Autodesk Inventor part; units mm, degrees
ref_plane "YZ Plane" through (0, 0, 0) normal (1, 0, 0) x (0, 1, 0)
ref_plane "XZ Plane" through (0, 0, 0) normal (0, 1, 0) x (-1, 0, 0)
ref_plane "XY Plane" through (0, 0, 0) normal (0, 0, 1) x (1, 0, 0)
sketch "スケッチ1" plane through (0, 0, 0) normal (0, 1, 0) x (-1, 0, 0)
  line L0 (-6, -13) -> (6, -13)
  line L1 (6, -13) -> (6, 13)
  line L2 (6, 13) -> (-6, 13)
  line L3 (-6, 13) -> (-6, -13)
  line L4 (-6, -13) -> (6, 13) construction
  line L5 (6, -13) -> (-6, 13) construction
  line L6 (6, 13) -> (-6, 13)
  line L7 (-6, 13) -> (-6, 5)
  line L8 (-6, 5) -> (6, 5)
  line L9 (6, 5) -> (6, 13)
  point P0 (0, 0)
  point P1 (0, 13)
  point P2 (-6, 13)
  point P3 (6, 5)
  dimension "d0" = 12
  dimension "d1" = 26
  dimension "d26" = 12
  dimension "d27" = 8
extrude "押し出し1" add sketch "スケッチ1" against normal blind 3 contours L3 L8 L1 L0
sketch "スケッチ5" plane through (0, 0, 0) normal (1, 0, 0) x (0, 1, 0)
  line L0 (-3, 5) -> (-3, -13)
  line L1 (-3, 5) -> (-3, 13)
  line L2 (-1.6051, 5) -> (-12.6984, 24.2141)
  line L3 (-12.6984, 24.2141) -> (-17.6984, 24.2141)
  line L4 (-16.3866, 0) -> (-3, 0)
  line L5 (0, 5) -> (-3, 5)
  line L6 (-17.6984, 24.2141) -> (-22.1813, 21.6259)
  line L7 (-22.1813, 21.6259) -> (-16.3866, 0)
  line L8 (-12.6984, 24.2141) -> (-8.3683, 26.7141) construction
  line L9 (-8.3683, 26.7141) -> (-7.6183, 25.4151) construction
  circle A0 centre (-7.6183, 25.4151) radius 1 construction
  line L10 (36.5, 48) -> (-6.3683, 23.25) construction
  line L11 (0, 13) -> (36.5, 13) construction
  line L12 (0, -13) -> (0, 5)
  line L13 (-3, 5) -> (-1.6051, 5)
  point P0 (0, 0)
  dimension "d28" = 8
  dimension "d29" = 120
  dimension "d31" = 5
  dimension "d32" = 5
  dimension "d35" = 5
  dimension "d36" = 150
  dimension "d37" = 75
  dimension "d47" = 5
  dimension "d48" = 1.5
  dimension "d49" = 2
  dimension "d50" = 2.5
  dimension "d51" = 49.5
  dimension "d53" = 8
  dimension "d54" = 36.5
  dimension "d55" = 35
extrude "押し出し5" add sketch "スケッチ5" against normal blind 4
sketch "スケッチ6" plane through (-4, 0, 0) normal (-1, 0, 0) x (0, 0, 1)
  line L0 (0, -3) -> (0, -16.3866)
  line L1 (0, -16.3866) -> (21.6259, -22.1813)
  line L2 (21.6259, -22.1813) -> (24.2141, -17.6984)
  line L3 (24.2141, -17.6984) -> (24.2141, -12.6984)
  line L4 (24.2141, -12.6984) -> (5, -1.6051)
  line L5 (0, -3) -> (5, -3)
  line L6 (19.884, -10.1984) -> (14.1259, -20.1716)
  line L7 (24.2141, -12.6984) -> (5.604, -1.9538)
  line L8 (5, -3) -> (5, -1.6051)
  point P0 (0, 0)
  dimension "d38" = 5
extrude "押し出し6" add sketch "スケッチ6" along normal blind 6 contours L6 L4 L3 L2 L1
mirror "ミラー3" about plane through (0, -11.8932, 12.1071) normal (1, 0, 0) of "押し出し5", "押し出し6"
sketch "スケッチ7" plane through (0, 0, 0) normal (0, 1, 0) x (1, 0, 0)
  circle A0 centre (4, -3) radius 1
  circle A1 centre (-4, 11) radius 1
  circle A2 centre (0, 0) radius 0.8
  circle A3 centre (0, 8) radius 0.8
  circle A4 centre (-4, 4) radius 0.8
  circle A5 centre (4, 4) radius 0.8
  circle A6 centre (4, 11) radius 1
  circle A7 centre (-4, -3) radius 1
  line L0 (6, -8) -> (6, -10)
  line L1 (30, -13) -> (9, -13)
  line L2 (33, -9.25) -> (33, -10)
  arc A8 (30, 6.25) -> (30, -6.25) centre (30, 0) ccw
  line L3 (33, 10) -> (33, 9.25)
  line L4 (-30, 13) -> (30, 13)
  line L5 (-33, -10) -> (-33, -9.25)
  arc A9 (-30, -6.25) -> (-30, 6.25) centre (-30, 0) ccw
  line L6 (-33, 9.25) -> (-33, 10)
  line L7 (-9, -13) -> (-30, -13)
  line L8 (-6, -10) -> (-6, -8)
  line L9 (-3, -5) -> (3, -5)
  line L10 (21.75, 7.5) -> (21.75, -7.5)
  line L11 (18.75, -10.5) -> (14, -10.5)
  line L12 (11, -7.5) -> (11, 7.5)
  line L13 (14, 10.5) -> (18.75, 10.5)
  circle A10 centre (9, 10.5) radius 0.85
  circle A11 centre (30, -10.5) radius 0.85
  circle A12 centre (-30, -10.5) radius 0.85
  circle A13 centre (-9, 10.5) radius 0.85
  circle A14 centre (-30, 10.5) radius 0.85
  circle A15 centre (-9, -10.5) radius 0.85
  circle A16 centre (9, -10.5) radius 0.85
  circle A17 centre (30, 10.5) radius 0.85
  line L14 (-11, 7.5) -> (-11, -7.5)
  line L15 (-14, -10.5) -> (-18.75, -10.5)
  line L16 (-21.75, -7.5) -> (-21.75, 7.5)
  line L17 (-18.75, 10.5) -> (-14, 10.5)
  arc A18 (-30, 13) -> (-33, 10) centre (-30, 10) ccw
  arc A19 (-33, 9.25) -> (-30, 6.25) centre (-30, 9.25) ccw
  arc A20 (-30, -6.25) -> (-33, -9.25) centre (-30, -9.25) ccw
  arc A21 (-33, -10) -> (-30, -13) centre (-30, -10) ccw
  arc A22 (-9, -13) -> (-6, -10) centre (-9, -10) ccw
  arc A23 (-3, -5) -> (-6, -8) centre (-3, -8) ccw
  arc A24 (6, -8) -> (3, -5) centre (3, -8) ccw
  arc A25 (6, -10) -> (9, -13) centre (9, -10) ccw
  arc A26 (30, -13) -> (33, -10) centre (30, -10) ccw
  arc A27 (33, -9.25) -> (30, -6.25) centre (30, -9.25) ccw
  arc A28 (30, 6.25) -> (33, 9.25) centre (30, 9.25) ccw
  arc A29 (33, 10) -> (30, 13) centre (30, 10) ccw
  arc A30 (-14, -10.5) -> (-11, -7.5) centre (-14, -7.5) ccw
  arc A31 (-21.75, -7.5) -> (-18.75, -10.5) centre (-18.75, -7.5) ccw
  arc A32 (-18.75, 10.5) -> (-21.75, 7.5) centre (-18.75, 7.5) ccw
  arc A33 (-11, 7.5) -> (-14, 10.5) centre (-14, 7.5) ccw
  arc A34 (18.75, -10.5) -> (21.75, -7.5) centre (18.75, -7.5) ccw
  arc A35 (11, -7.5) -> (14, -10.5) centre (14, -7.5) ccw
  arc A36 (14, 10.5) -> (11, 7.5) centre (14, 7.5) ccw
  arc A37 (21.75, 7.5) -> (18.75, 10.5) centre (18.75, 7.5) ccw
  point P0 (0, 0)
extrude "押し出し7" cut sketch "スケッチ7" against normal up to surface (3 mm away) contours A0 | A1 | A2 | A3 | A4 | A5 | A6 | A7
sketch "スケッチ8" plane through (0, -3, 0) normal (0, -1, 0) x (1, 0, 0)
  line L0 (-6, 5) -> (6, 5)
  line L1 (-6, -13) -> (-6, 5)
  line L2 (6, -13) -> (-6, -13)
  line L3 (6, 5) -> (6, -13)
  point P0 (0, 0)
extrude "押し出し8" add sketch "スケッチ8" along normal blind 23
sketch "スケッチ9" plane through (0, -26, 0) normal (0, -1, 0) x (1, 0, 0)
  circle A0 centre (-4, 3) radius 1
  circle A1 centre (4, 3) radius 1
  circle A2 centre (4, -11) radius 1
  circle A3 centre (4, -11) radius 1
  circle A4 centre (-4, -11) radius 1
  circle A5 centre (-4, -11) radius 1
  point P0 (0, 0)
extrude "押し出し9" cut sketch "スケッチ9" against normal blind 7
sketch "スケッチ10" plane through (10, -17.6984, 24.2141) normal (1, 0, 0) x (0, 0, -1)
  circle A0 centre (2, 2.5) radius 1 construction
  circle A1 centre (7.0529, -1.216) radius 1 construction
  circle A2 centre (2, 2.5) radius 0.8
  circle A3 centre (7.0529, -1.216) radius 0.8
  point P0 (24.2141, 17.6984)
  dimension "d56" = 1.6
  dimension "d57" = 1.6
extrude "押し出し10" cut sketch "スケッチ10" against normal through all
sketch "スケッチ11" plane through (6, 0, 5) normal (1, 0, 0) x (0, 0, -1)
  line L0 (18, 0) -> (18, -26)
  line L1 (18, -11) -> (20, -11)
  line L2 (20, -11) -> (20, -26)
  line L3 (20, -26) -> (18, -26)
  line L4 (18, -26) -> (18, -11)
  line L5 (18, -26) -> (0, -26)
  point P0 (5, 0)
  dimension "d60" = 15
  dimension "d61" = 2
extrude "押し出し11" add sketch "スケッチ11" against normal up to surface (12 mm away)
sketch "スケッチ12" plane through (0, 0, 0) normal (1, 0, 0) x (0, 1, 0)
  line L0 (-26, -15) -> (-11, -15)
  line L1 (-11, -15) -> (-26, -15)
  line L2 (-26, -15) -> (-26, -19)
  line L3 (-26, -19) -> (-11, -19)
  line L4 (-11, -19) -> (-11, -15)
  line L5 (-22, -19) -> (-26, -19)
  line L6 (-26, -19) -> (-26, -37)
  line L7 (-26, -37) -> (-22, -37)
  line L8 (-22, -37) -> (-22, -19)
  line L9 (-26, 5) -> (-26, -15)
  point P0 (0, 0)
  dimension "d64" = 4
  dimension "d65" = 4
  dimension "d66" = 18
extrude "押し出し12" add sketch "スケッチ12" against normal blind 19
mirror "ミラー4" about plane through (0, -18.5, -26) normal (1, 0, 0) of "押し出し12"
sketch "スケッチ13" plane through (-6, -11, -13) normal (0, 1, 0) x (1, 0, 0)
  line L0 (-15, 6) -> (27, 6)
  line L1 (27, 6) -> (27, 2)
  line L2 (27, 2) -> (-15, 2)
  line L3 (-15, 2) -> (-15, 6)
  line L4 (0, 2) -> (-13, 2)
  line L5 (-13, 6) -> (25, 6)
  line L6 (25, 2) -> (25, 6)
  line L7 (-15, 2) -> (-13, 2)
  line L8 (-13, 2) -> (-13, 17)
  line L9 (-13, 17) -> (-15, 17)
  line L10 (-15, 17) -> (-15, 2)
  line L11 (27, 2) -> (25, 2)
  line L12 (25, 2) -> (25, 17)
  line L13 (25, 17) -> (27, 17)
  line L14 (27, 17) -> (27, 2)
  line L15 (-13, 2) -> (-13, 6)
  point P0 (6, -13)
  point P1 (25, 6)
  point P2 (27, 6)
  point P3 (-13, 2)
  point P4 (-15, 6)
  dimension "d75" = 2
  dimension "d76" = 2
  dimension "d77" = 15
extrude "押し出し13" add sketch "スケッチ13" along normal blind 30 contours L10 L9 L8 L0 | L0 L8 L2 L3 | L12 L13 L14 L0 | L0 L1 L2 L6
sketch "スケッチ14" plane through (-6, -11, -13) normal (0, 1, 0) x (1, 0, 0)
  line L0 (0, 2) -> (0, 0)
  line L1 (12, 0) -> (0, 0)
  line L2 (12, 2) -> (12, 0)
  line L3 (12, 2) -> (25, 2)
  line L4 (25, 2) -> (25, 6)
  line L5 (-13, 6) -> (25, 6)
  line L6 (-13, 2) -> (-13, 6)
  line L7 (0, 2) -> (-13, 2)
  point P0 (6, -13)
extrude "押し出し14" add sketch "スケッチ14" along normal blind 5
fillet "フィレット1" radius 10 2 edges at (-19, -6, -17) (19, -6, -17)
sketch "スケッチ16" plane through (21, -11, -15) normal (1, 0, 0) x (0, 0, -1)
  line L0 (15, 30) -> (0, 30)
  line L1 (7.5, 30) -> (15, 17.0096)
  line L2 (15, 0) -> (15, 30)
  point P0 (-15, 11)
  dimension "d85" = 120
extrude "押し出し16" cut sketch "スケッチ16" along normal through all both and the other way through all
sketch "スケッチ17" plane through (19, -26, -37) normal (1, 0, 0) x (0, 0, -1)
  circle A0 centre (-2, 4) radius 1.6
  point P0 (-37, 26)
extrude "押し出し17" cut sketch "スケッチ17" against normal through all
sketch "スケッチ18" plane through (19, -26, -37) normal (1, 0, 0) x (0, 0, -1)
  circle A0 centre (-20, 10) radius 0.8
  circle A1 centre (-20, 2) radius 0.8
  circle A2 centre (-8, 2) radius 0.8
  line L0 (-22, 0) -> (-22, 15)
  line L1 (0, 0) -> (-22, 0)
  point P0 (-37, 26)
  dimension "d90" = 1.6
  dimension "d91" = 1.6
  dimension "d92" = 1.6
  dimension "d93" = 2
  dimension "d94" = 2
  dimension "d95" = 8
  dimension "d96" = 12
extrude "押し出し18" cut sketch "スケッチ18" against normal blind 5
mirror "ミラー5" about plane through (0, 0, 0) normal (1, 0, 0) of "押し出し18"
equation "\"d76\" = d75"
properties part number "hipjoint_middle"
Geometry check sheet. Reference: the model listing, model coordinates, mm. A direction names the side the tool comes from. Round coordinates to 2 decimals unless told otherwise and drop trailing zeros. Write each loop counter-clockwise with the first axis right and the second up, starting at its lowest first coordinate (ties: lowest second). Pieces come first, ordered by that corner, then holes. Notation, with made-up numbers: (50, 57) - (102, 57) arc R15 cw to (102, 61) - close; hole circle Ø7 at (77.25, 80.5). An arc over 180 degrees is marked (long way). Write each question's results on one line, items separated by ' | '.
(1) Thickness scan on probe 1 along Z at (x, y) = (-4, -0.9); probe 2 along X at (y, z) = (7.5, -29); probe 3 along X at (y, z) = (-1, 0). Record the ranges inside material, lowest first. Write a range as from..to.
Computed:
probe 1: z = -13..-12, -10..-4.8, -3.2..2, 4..5 | probe 2: x = -21..-19, 19..21 | probe 3: x = -6..-0.8, 0.8..6
(2) Sectioned sample at D-D, the plane z = -23.5. Enter the section's corners in (x, y).
Computed:
outline: (-21, -11) - (-19, -11) - (-19, 17.27) - (-21, 17.27) - close; (-19, -26) - (19, -26) - (19, -22) - (-19, -22) - close; (19, -11) - (21, -11) - (21, 17.27) - (19, 17.27) - close
(3) Sectioned sample at C-C, the plane z = -11. Enter the section's corners in (x, y).
Computed:
outline: (-6, -26) - (-5, -26) - (-5, -19) - (-3, -19) - (-3, -26) - (3, -26) - (3, -19) - (5, -19) - (5, -26) - (6, -26) - (6, 0) - (5, 0) - (5, -3) - (3, -3) - (3, 0) - (-3, 0) - (-3, -3) - (-5, -3) - (-5, 0) - (-6, 0) - close
(4) Sectioned sample at B-B, the plane y = 8.5. Enter the section's corners in (x, z), plus the area to 3 significant figures.
Computed:
outline: (-21, -28.56) - (-19, -28.56) - (-19, -15) - (-21, -15) - close; (19, -28.56) - (21, -28.56) - (21, -15) - (19, -15) - close | area: 54.2 mm^2
(5) Sectioned sample at A-A, the plane x = 8. Enter the section's corners in (y, z).
Computed:
outline: (-26, -37) - (-22, -37) - (-22, -36.6) arc R1.6 cw to (-22, -33.4) - (-22, -19) - (-6, -19) - (-6, -15) - (-26, -15) - close; (-22.18, 21.63) - (-20.17, 14.13) - (-10.2, 19.88) - (-12.7, 24.21) - (-17.7, 24.21) - close; hole circle Ø1.6 at (-18.91, 17.16); hole circle Ø1.6 at (-15.2, 22.21)
(6) Depth check by flat-ended pin: pin 1 Ø6 at (x, y) = (14, -12) entering from -Z; pin 2 Ø4.5 at (y, z) = (-7.5, 12.5) entering from -X; pin 3 Ø1.2 at (x, z) = (-4, -11) entering from -Y. Enter the tip coordinate at first touch or a pass-through.
Computed:
pin 1: stops at z = -19 | pin 2: stops at x = -4 | pin 3: stops at y = -19
(7) Set-up check for faces 1 (the face through (0, -3, -13)), 2 (the face through (-15.99, -3.15, -17.03)), 3 (the face through (4, -3, 3)): record each of +Z, -Z, +X, -X, +Y, -Y from which the full face is reachable in a straight line by a thin tool's end or side.
Computed:
face 1: -Z, +X, -X, +Y | face 2: +Z, -Z, +Y | face 3: +Y
(8) Draft check along Y on faces 4 (the face through (16.535, -24.306, -29.739)), 5 (the face through (-6, -13, -5)), 6 (the face through (6.958, -15.255, 16.965)). Enter one of: pulls with the +Y half, pulls with the -Y half, needs draft (parallel to the pull), parting line crosses it, or undercut.
Computed:
face 4: undercut | face 5: needs draft | face 6: pulls with the +Y half
